Could you check a few things on this drawing? It's one solid part, dimensions in mm from its lowest x, y, z. A direction names the side the tool comes from. Round coordinates to 2 decimals unless told otherwise and drop trailing zeros. Write each loop counter-clockwise with the first axis right and the second up, starting at its lowest first coordinate (ties: lowest second). Pieces come first, ordered by that corner, then holes. Notation, with made-up numbers: (34.5, 57.5) -> (51.5, 57.5) arc R7 cw to (51.5, 70.5) -> close; hole circle Ø7 at (38.25, 78.5). An arc over 180 degrees is marked (long way). Return JSON: item names as keys, results as strings.
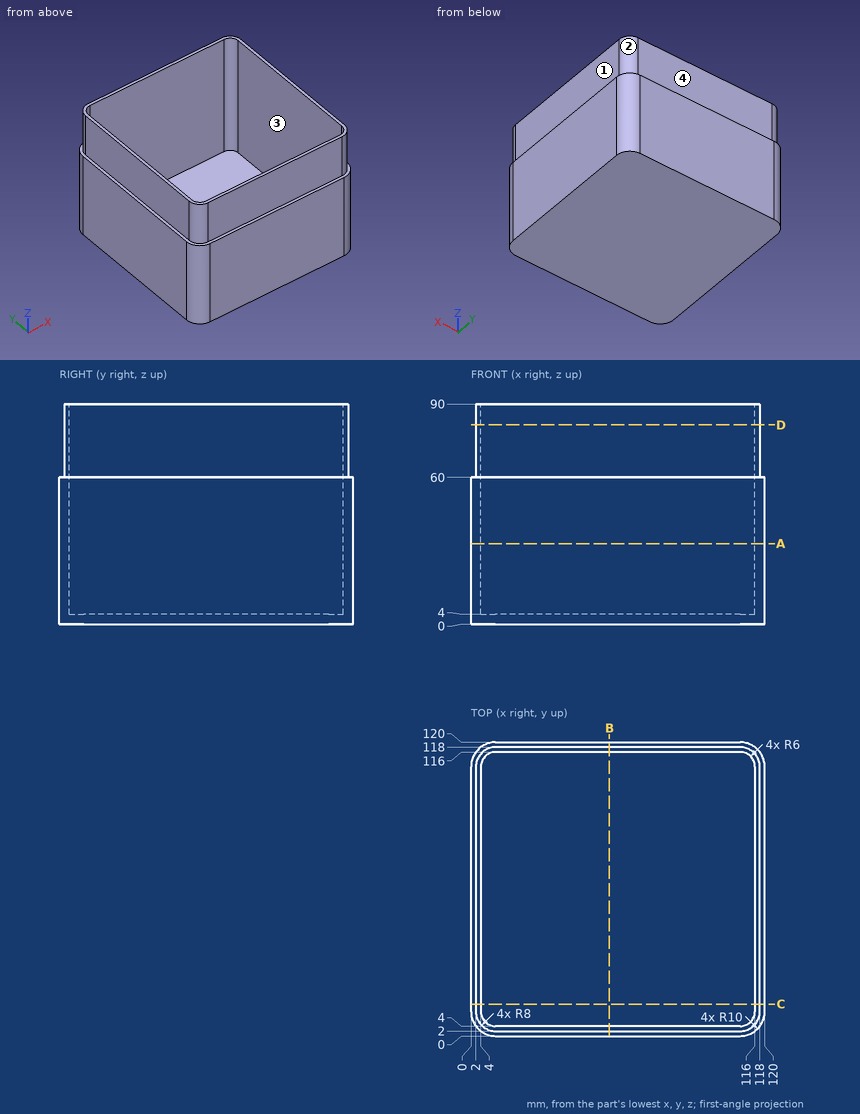
1) I want a section at A-A, the plane z = 33. Please give me the cut outline in (x, y), and give its area (3 significant figures).
Return value:
{"outline": "(0, 10) arc R10 ccw to (10, 0) -> (110, 0) arc R10 ccw to (120, 10) -> (120, 110) arc R10 ccw to (110, 120) -> (10, 120) arc R10 ccw to (0, 110) -> close; hole (4, 10) arc R6 ccw to (10, 4) -> (110, 4) arc R6 ccw to (116, 10) -> (116, 110) arc R6 ccw to (110, 116) -> (10, 116) arc R6 ccw to (4, 110) -> close", "area": "1,800 mm²"}
2) I want a section at D-D, the plane z = 81.5. Please give me the cut outline in (x, y).
Return value:
{"outline": "(2, 10) arc R8 ccw to (10, 2) -> (110, 2) arc R8 ccw to (118, 10) -> (118, 110) arc R8 ccw to (110, 118) -> (10, 118) arc R8 ccw to (2, 110) -> close; hole (4, 10) arc R6 ccw to (10, 4) -> (110, 4) arc R6 ccw to (116, 10) -> (116, 110) arc R6 ccw to (110, 116) -> (10, 116) arc R6 ccw to (4, 110) -> close"}
3) For the marked faces 1, 2, 3 and 4, which set-ups out of +Z, -Z, +X, -X, +Y, -Y let a thin tool reach every point of the face, with its end or its side?
Return value:
{"face 1": "+Z, +X, +Y, -Y", "face 2": "+Z, +X, +Y", "face 3": "+Z", "face 4": "+Z, +X, -X, +Y"}
4) Will these pins go through, and if not, where does the flat tip stop? pin 1 Ø9 at (x, z) = (62.5, 75.5) entering from +Y; pin 2 Ø8 at (x, z) = (40.5, 75) entering from -Y; pin 3 Ø15 at (y, z) = (56, 72) entering from -X.
Return value:
{"pin 1": "y = 118", "pin 2": "y = 2", "pin 3": "x = 2"}
5) I want a section at B-B, the plane x = 56.5. Please give me the cut outline in (y, z).
Return value:
{"outline": "(0, 0) -> (120, 0) -> (120, 60) -> (118, 60) -> (118, 90) -> (116, 90) -> (116, 4) -> (4, 4) -> (4, 90) -> (2, 90) -> (2, 60) -> (0, 60) -> close"}
6) If I drill on probe 1 along X at (y, z) = (102, 35.5); probe 2 along Y at (x, z) = (71, 73.5), over which ranges is the centre line in solid material (lowest first)? Write a range as [from, to].
Return value:
{"probe 1": "[0, 4], [116, 120]", "probe 2": "[2, 4], [116, 118]"}
